The model under review builds one solid part; all positions refer to its coordinate system, in mm. A direction names the side the tool comes from. Coordinates: 2 decimals unless noted, no trailing zeros. Write each loop counter-clockwise with the first axis right and the second up, starting at its lowest first coordinate (ties: lowest second). Pieces come first, ordered by that corner, then holes. Notation, with made-up numbers: (27, 54.5) -> (33, 54.5) arc R25 ccw to (33, 74.5) -> close; hole circle Ø7 at (41.5, 76.5). An arc over 180 degrees is marked (long way). Write each question's results on one line, items separated by ' | '.
```python
from build123d import *

# Parameters (mm, degrees)
ESBO_O1_W                  = 125
ESBO_O1_H                  = 40
BASE_DEPTH                 = 7
ESBO_O2_W                  = 5
ESBO_O2_H                  = 40
SUPORTE_LATERAL_DEPTH      = 20
ESBO_O3_R                  = 1.625
FURO_MOTOR_DEPTH           = 7
ESBO_O4_W                  = 6
ESBO_O4_H                  = 10
CORTE_EXTRUS_O2_DEPTH      = 69.60211367
CORTE_EXTRUS_O3_DEPTH      = 69.60211367
CORTE_EXTRUS_O3_DEPTH_BACK = 69.60211367
ESBO_O5_R                  = 2.5
CORTE_EXTRUS_O4_DEPTH      = 69.60211367
CORTE_EXTRUS_O5_DEPTH      = 2.5
ESBO_O9_R                  = 2.5
CORTE_EXTRUS_O6_DEPTH      = 70.372184628
CORTE_EXTRUS_O7_DEPTH      = 125.615408357
CORTE_EXTRUS_O7_DEPTH_BACK = 125.615408357
ESBO_O10_R                 = 1.625
FILETE1_R                  = 2


with BuildPart() as part:
    # Esboço1 → base (new body)
    with BuildSketch(Plane(origin=(0, 0, 0), x_dir=(1, 0, 0), z_dir=(0, 1, 0))):
        Rectangle(ESBO_O1_W, ESBO_O1_H)
    extrude(amount=BASE_DEPTH)

    # Esboço2 → suporte lateral (add)
    with BuildSketch(Plane(origin=(0, 7, 0), x_dir=(1, 0, 0), z_dir=(0, 1, 0))):
        with Locations((60, 0)):
            Rectangle(ESBO_O2_W, ESBO_O2_H)
        with Locations((-60, 0)):
            Rectangle(ESBO_O2_W, ESBO_O2_H)
    extrude(amount=SUPORTE_LATERAL_DEPTH)

    # Esboço3 → furo motor (cut)
    with BuildSketch(Plane(origin=(0, 7, 0), x_dir=(1, 0, 0), z_dir=(0, 1, 0))):
        with Locations(Location((-40.5, 0, 0), (0, 0, 270))):
            Circle(ESBO_O3_R)
        with Locations(Location((-40.5, 11.5, 0), (0, 0, 270))):
            Circle(ESBO_O3_R)
        with Locations(Location((-40.5, -11.5, 0), (0, 0, 270))):
            Circle(ESBO_O3_R)
        with Locations(Location((40.5, 11.5, 0), (0, 0, 270))):
            Circle(ESBO_O3_R)
        with Locations(Location((40.5, 0, 0), (0, 0, 270))):
            Circle(ESBO_O3_R)
        with Locations(Location((40.5, -11.5, 0), (0, 0, 270))):
            Circle(ESBO_O3_R)
    extrude(amount=-FURO_MOTOR_DEPTH, mode=Mode.SUBTRACT)

    # Esboço4 → Corte-extrusão2 (cut, through all)
    with BuildSketch(Plane(origin=(0, 7, 0), x_dir=(1, 0, 0), z_dir=(0, 1, 0))):
        with Locations((25, 0)):
            Rectangle(ESBO_O4_W, ESBO_O4_H)
        with Locations((-25, 0)):
            Rectangle(ESBO_O4_W, ESBO_O4_H)
    extrude(amount=-CORTE_EXTRUS_O2_DEPTH, mode=Mode.SUBTRACT)

    # Esboço5 → Corte-extrusão3 (cut, two sides: drawn at the far end of the back side and taken through both)
    with BuildSketch(Plane(origin=(0, 7, 0), x_dir=(1, 0, 0), z_dir=(0, 1, 0)).offset(-CORTE_EXTRUS_O3_DEPTH_BACK)):
        with Locations(Location((0, 9, 0), (0, 0, 270))):
            Circle(ESBO_O5_R)
        with Locations(Location((0, -9, 0), (0, 0, 270))):
            Circle(ESBO_O5_R)
    extrude(amount=CORTE_EXTRUS_O3_DEPTH + CORTE_EXTRUS_O3_DEPTH_BACK, mode=Mode.SUBTRACT)

    # Esboço7 → Corte-extrusão4 (cut, through all)
    with BuildSketch(Plane(origin=(0, 7, 0), x_dir=(1, 0, 0), z_dir=(0, 1, 0))):
        with BuildLine():
            ThreePointArc((52, 6), (49.75, 3.75), (47.5, 6))
            Line((47.5, 6), (47.5, 12))
            ThreePointArc((47.5, 12), (49.75, 14.25), (52, 12))
            Line((52, 12), (52, 6))
        make_face()
        with BuildLine():
            ThreePointArc((47.5, -6), (49.75, -3.75), (52, -6))
            Line((52, -6), (52, -12))
            ThreePointArc((52, -12), (49.75, -14.25), (47.5, -12))
            Line((47.5, -12), (47.5, -6))
        make_face()
        with BuildLine():
            Line((-52, -6), (-52, -12))
            ThreePointArc((-52, -12), (-49.75, -14.25), (-47.5, -12))
            Line((-47.5, -12), (-47.5, -6))
            ThreePointArc((-47.5, -6), (-49.75, -3.75), (-52, -6))
        make_face()
        with BuildLine():
            ThreePointArc((-47.5, 12), (-49.75, 14.25), (-52, 12))
            Line((-52, 12), (-52, 6))
            ThreePointArc((-52, 6), (-49.75, 3.75), (-47.5, 6))
            Line((-47.5, 6), (-47.5, 12))
        make_face()
    extrude(amount=-CORTE_EXTRUS_O4_DEPTH, mode=Mode.SUBTRACT)

    # Esboço8 → Corte-extrusão5 (cut)
    with BuildSketch(Plane(origin=(0, 7, 0), x_dir=(1, 0, 0), z_dir=(0, 1, 0))):
        with BuildLine():
            Line((4.25, 9), (4.25, -9))
            ThreePointArc((4.25, -9), (0, -13.25), (-4.25, -9))
            Line((-4.25, -9), (-4.25, 9))
            ThreePointArc((-4.25, 9), (0, 13.25), (4.25, 9))
        make_face()
    extrude(amount=-CORTE_EXTRUS_O5_DEPTH, mode=Mode.SUBTRACT)

    # Esboço9 → Corte-extrusão6 (cut, through all)
    with BuildSketch(Plane(origin=(0, 4.5, 0), x_dir=(1, 0, 0), z_dir=(0, 1, 0))):
        with Locations(Location((0, 0, 0), (0, 0, 270))):
            Circle(ESBO_O9_R)
    extrude(amount=-CORTE_EXTRUS_O6_DEPTH, mode=Mode.SUBTRACT)

    # Esboço10 → Corte-extrusão7 (cut, two sides: drawn at the far end of the back side and taken through both)
    with BuildSketch(Plane.ZY.offset(-57.5).offset(-CORTE_EXTRUS_O7_DEPTH_BACK)):
        with Locations((-12, 21.8)):
            Circle(ESBO_O10_R)
        with Locations((0, 21.8)):
            Circle(ESBO_O10_R)
        with Locations((12, 21.8)):
            Circle(ESBO_O10_R)
        with Locations((-12, 12.2)):
            Circle(ESBO_O10_R)
        with Locations((0, 12.2)):
            Circle(ESBO_O10_R)
        with Locations((12, 12.2)):
            Circle(ESBO_O10_R)
    extrude(amount=CORTE_EXTRUS_O7_DEPTH + CORTE_EXTRUS_O7_DEPTH_BACK, mode=Mode.SUBTRACT)

    # Filete1
    filete1_edges = [part.edges().sort_by_distance(p)[0] for p in [
        (22, 3.5, 5),
        (22, 3.5, -5),
        (28, 3.5, -5),
        (28, 3.5, 5),
        (-28, 3.5, 5),
        (-28, 3.5, -5),
        (-22, 3.5, -5),
        (-22, 3.5, 5),
    ]]
    fillet(filete1_edges, radius=FILETE1_R)


solid = part.part
```
Q1. Machinability: for faces 3 (the cylindrical face through (0.09, 5.77, 13.25)), 4 (the cylindrical face through (60.04, 20.81, -1.29)), 5 (the flat face through (-28, 4, 0)), which of the approach directions +Z, -Z, +X, -X, +Y, -Y give a long, thin tool a straight path to every point of the face, cutting with its end or side? Answer none if there is none.
Solution:
face 3: +Y | face 4: +X, -X | face 5: +Y, -Y
Q2. Add section C-C (z = 0). Count the separate pieces of the cut face and the enclosed holes in it, plus the area to 3 significant figures.
Solution:
separate pieces: 10 | enclosed holes: 0 | area: 837 mm²
Q3. Add section D-D (x = -31.5). Write out the cut boundary in (y, z).
Solution:
outline: (0, -20) -> (7, -20) -> (7, 20) -> (0, 20) -> close
Q4. Draft analysis for pull direction Z (two halves, no side actions). For faces 1 (the flat face through (-62.5, 10, 0)), 2 (the cylindrical face through (-59.965, 21.871, -13.623)), state which applies: pulls with the +Z half, pulls with the -Z half, needs draft (parallel to the pull), parting line crosses it, or undercut.
Solution:
face 1: needs draft | face 2: undercut
Q5. For line 1 (Y direction, x = 59, z = 12) (3 decimals); line 2 (X direction, y = 5.5, z = -3); line 3 (Z direction, x = 61.1, y = 12.2) (3 decimals), list the stretches that pass through material, from the lowest coordinate up. Write a range as from..to.
Solution:
line 1: 0..10.575, 13.825..20.175, 23.425..27 | line 2: -62.5..-28, -22..-4.25, 4.25..22, 28..62.5 | line 3: -20..-13.625, -10.375..-1.625, 1.625..10.375, 13.625..20
Q6. Add section B-B (y = 25.25). Write out the cut boundary in (x, z).
Solution:
outline: (-62.5, -20) -> (-57.5, -20) -> (-57.5, 20) -> (-62.5, 20) -> close; (57.5, -20) -> (62.5, -20) -> (62.5, 20) -> (57.5, 20) -> close
Q7. Clearance check with flat-ended pins moving along their axes: P1, Ø4, axis at x = 0, z = -9, coming from the -Y side; P2, Ø4, axis at x = 46, z = -0.5, coming from the +Y side; P3, Ø4, axis at x = 1, z = 6.5, coming from the +Y side. State where each tip first meets the part, or that it passes through.
Solution:
P1: through | P2: y = 7 | P3: y = 4.5
Q8. Add section A-A (x = 40.5). Write out the cut boundary in (y, z) (3 decimals).
Solution:
outline: (0, -20) -> (7, -20) -> (7, -13.125) -> (0, -13.125) -> close; (0, -9.875) -> (7, -9.875) -> (7, -1.625) -> (0, -1.625) -> close; (0, 1.625) -> (7, 1.625) -> (7, 9.875) -> (0, 9.875) -> close; (0, 13.125) -> (7, 13.125) -> (7, 20) -> (0, 20) -> close
